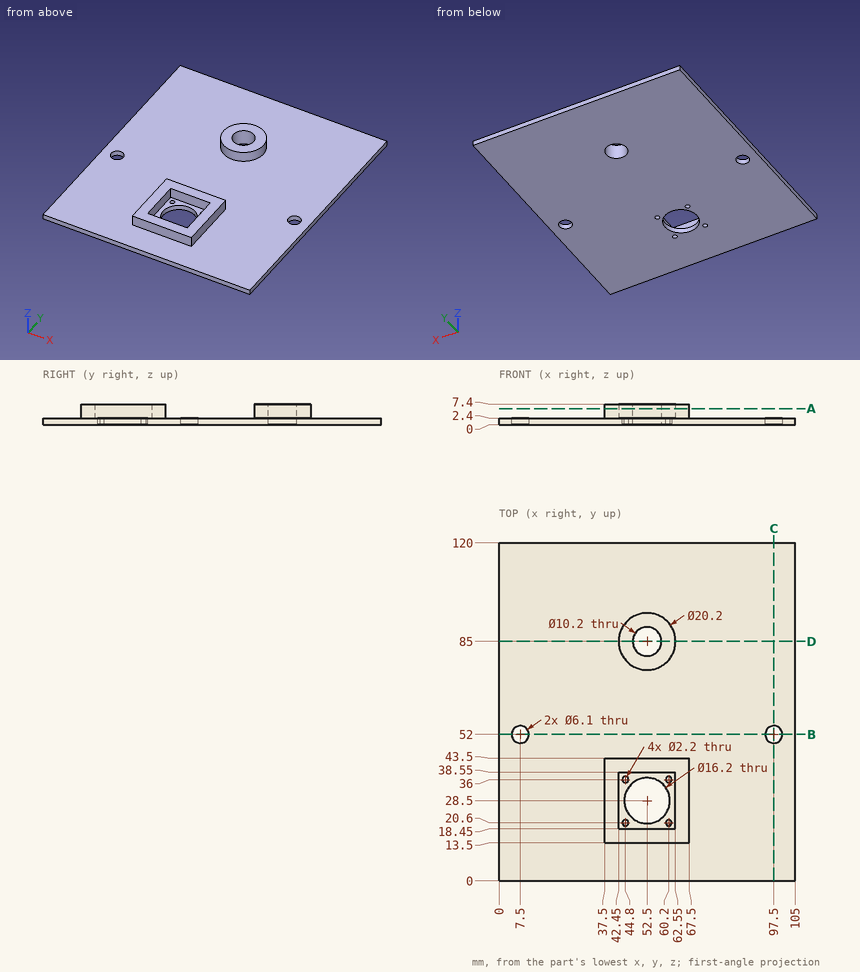
Geometry check sheet. Reference: drawing and pictorial views, mm from the part's lowest x, y, z. Coordinates: 2 decimals unless noted, no trailing zeros. Order: outer loops, then holes, each group sorted by start corner. A loop starts at its lowest first (then second) coordinate and runs counter-clockwise, first axis right, second up. Notation, with made-up numbers: (79.5, 53.25) - (94.5, 53.25) arc R38 ccw to (94.5, 92.25) - close; hole circle Ø10 at (35, -27.5). An arc over 180 degrees is marked (long way). Answer in a Markdown table with one row per item. Add a question column.
1) Cross-section at A-A, the plane z = 5.75. Record the cut outline in (x, y).
2) Cross-section at B-B, the plane y = 52. Record the cut outline in (x, z).
3) Gauge pin test, flat ends, axial feed: P1, Ø2.5, axis at x = 55, z = 4, coming from the +Y side; P2, Ø1, axis at x = 27.5, y = 87, coming from the +Z side; P3, Ø2.5, axis at y = 32.5, z = 5, coming from the -X side. Record the tip position at first contact, or that the pin passes through.
4) Material ranges on line 1 along Y through (x, z) = (52.5, 1.7); line 2 along Y through (x, z) = (52.5, 4); line 3 along X through (y, z) = (28, 2.5), recorded low to high. Write a range as [from, to].
5) Cross-section at D-D, the plane y = 85. Record the cut outline in (x, z).
6) Cross-section at C-C, the plane x = 97.5. Record the cut outline in (y, z).
Check result:
| question | item | result |
|---|---|---|
| 1 | outline | (37.5, 13.5) - (67.5, 13.5) - (67.5, 43.5) - (37.5, 43.5) - close; circle Ø20.2 at (52.5, 85); hole (42.45, 18.45) - (62.55, 18.45) - (62.55, 38.55) - (42.45, 38.55) - close; hole circle Ø10.2 at (52.5, 85) |
| 2 | outline | (0, 0) - (4.45, 0) - (4.45, 2.4) - (0, 2.4) - close; (10.55, 0) - (94.45, 0) - (94.45, 2.4) - (10.55, 2.4) - close; (100.55, 0) - (105, 0) - (105, 2.4) - (100.55, 2.4) - close |
| 3 | P1 | stops at y = 95.02 |
| 3 | P2 | stops at z = 2.4 |
| 3 | P3 | stops at x = 37.5 |
| 4 | line 1 | y = [0, 20.4], [36.6, 79.9], [90.1, 120] |
| 4 | line 2 | y = [13.5, 18.45], [38.55, 43.5], [74.9, 79.9], [90.1, 95.1] |
| 4 | line 3 | x = [37.5, 42.45], [62.55, 67.5] |
| 5 | outline | (0, 0) - (47.4, 0) - (47.4, 7.4) - (42.4, 7.4) - (42.4, 2.4) - (0, 2.4) - close; (57.6, 0) - (105, 0) - (105, 2.4) - (62.6, 2.4) - (62.6, 7.4) - (57.6, 7.4) - close |
| 6 | outline | (0, 0) - (48.95, 0) - (48.95, 2.4) - (0, 2.4) - close; (55.05, 0) - (120, 0) - (120, 2.4) - (55.05, 2.4) - close |
